from build123d import *

# Parameters (mm, degrees)
SKETCH_1_R      = 4
SKETCH_1_R_2    = 1.5
SKETCH_1_R_3    = 2
EXTRUDE_1_DEPTH = 2
SKETCH_2_R      = 1.5
EXTRUDE_2_DEPTH = 2
FILLET_2_R      = 2
SKETCH_3_R      = 2
EXTRUDE_3_DEPTH = 2
FILLET_3_R      = 2
FILLET_4_R      = 2


with BuildPart() as part:
    # 草图1 → 凸台-拉伸1 (new body)
    with BuildSketch(Plane.XY):
        with BuildLine():
            Line((-17, 18.75), (17, 18.75))
            ThreePointArc((17, 18.75), (18.414213562, 18.164213562), (19, 16.75))
            Line((19, 16.75), (19, 6.838490702))
            Line((19, 6.838490702), (20, 6.838490702))
            Line((20, 6.838490702), (20, 9.75))
            Line((20, 9.75), (27, 9.75))
            Line((27, 9.75), (29, 9.75))
            Line((29, 9.75), (29, 7.75))
            Line((29, 7.75), (29, -9.12411328))
            ThreePointArc((29, -9.12411328), (28.414213562, -10.538326843), (27, -11.12411328))
            Line((27, -11.12411328), (20, -11.12411328))
            Line((20, -11.12411328), (20, -16.75))
            Line((20, -16.75), (20, -18.75))
            Line((20, -18.75), (18, -18.75))
            Line((18, -18.75), (-18, -18.75))
            Line((-18, -18.75), (-20, -18.75))
            Line((-20, -18.75), (-20, -16.75))
            Line((-20, -16.75), (-20, -11.12411328))
            Line((-20, -11.12411328), (-27, -11.12411328))
            ThreePointArc((-27, -11.12411328), (-28.414213562, -10.538326843), (-29, -9.12411328))
            Line((-29, -9.12411328), (-29, 7.75))
            Line((-29, 7.75), (-29, 9.75))
            Line((-29, 9.75), (-27, 9.75))
            Line((-27, 9.75), (-20, 9.75))
            Line((-20, 9.75), (-20, 6.838490702))
            Line((-20, 6.838490702), (-19, 6.838490702))
            Line((-19, 6.838490702), (-19, 16.75))
            ThreePointArc((-19, 16.75), (-18.414213562, 18.164213562), (-17, 18.75))
        make_face()
        with Locations((0, -6.75)):
            Circle(SKETCH_1_R, mode=Mode.SUBTRACT)
        with Locations((-10.5, 3.75)):
            Circle(SKETCH_1_R, mode=Mode.SUBTRACT)
        with Locations((-7, -6.75)):
            Circle(SKETCH_1_R_2, mode=Mode.SUBTRACT)
        with Locations((0, 0.25)):
            Circle(SKETCH_1_R_2, mode=Mode.SUBTRACT)
        with Locations((7, -6.75)):
            Circle(SKETCH_1_R_2, mode=Mode.SUBTRACT)
        with Locations((0, -13.75)):
            Circle(SKETCH_1_R_2, mode=Mode.SUBTRACT)
        with Locations((-17.5, 3.75)):
            Circle(SKETCH_1_R_2, mode=Mode.SUBTRACT)
        with Locations((10.5, -3.25)):
            Circle(SKETCH_1_R_2, mode=Mode.SUBTRACT)
        with Locations((-10.5, 10.75)):
            Circle(SKETCH_1_R_2, mode=Mode.SUBTRACT)
        with Locations((-3.5, 3.75)):
            Circle(SKETCH_1_R_2, mode=Mode.SUBTRACT)
        with Locations((-10.5, -3.25)):
            Circle(SKETCH_1_R_2, mode=Mode.SUBTRACT)
        with Locations((17.5, 3.75)):
            Circle(SKETCH_1_R_2, mode=Mode.SUBTRACT)
        with Locations((3.5, 3.75)):
            Circle(SKETCH_1_R_2, mode=Mode.SUBTRACT)
        with Locations((10.5, 3.75)):
            Circle(SKETCH_1_R, mode=Mode.SUBTRACT)
        with Locations((10.5, 10.75)):
            Circle(SKETCH_1_R_2, mode=Mode.SUBTRACT)
        with Locations((-24.315, -6.25)):
            Circle(SKETCH_1_R_3, mode=Mode.SUBTRACT)
        with Locations((-24.315, 3.75)):
            Circle(SKETCH_1_R_3, mode=Mode.SUBTRACT)
        with Locations((24.315, 3.75)):
            Circle(SKETCH_1_R_3, mode=Mode.SUBTRACT)
        with Locations((24.315, -6.25)):
            Circle(SKETCH_1_R_3, mode=Mode.SUBTRACT)
    extrude(amount=EXTRUDE_1_DEPTH)

    # 草图2 → 凸台-拉伸2 (add)
    with BuildSketch(Plane.XZ.offset(18.75)):
        with BuildLine():
            Line((-20, 0), (20, 0))
            Line((20, 0), (20, 25))
            ThreePointArc((20, 25), (19.414213562, 26.414213562), (18, 27))
            Line((18, 27), (-18, 27))
            ThreePointArc((-18, 27), (-19.414213562, 26.414213562), (-20, 25))
            Line((-20, 25), (-20, 0))
        make_face()
        with Locations((9.7, 14)):
            Circle(SKETCH_2_R, mode=Mode.SUBTRACT)
        with Locations((-9.7, 14)):
            Circle(SKETCH_2_R, mode=Mode.SUBTRACT)
        with Locations((-2.7, 14)):
            Circle(SKETCH_2_R, mode=Mode.SUBTRACT)
        with Locations((16.7, 14)):
            Circle(SKETCH_2_R, mode=Mode.SUBTRACT)
        with Locations((9.7, 7)):
            Circle(SKETCH_2_R, mode=Mode.SUBTRACT)
        with Locations((2.7, 14)):
            Circle(SKETCH_2_R, mode=Mode.SUBTRACT)
        with Locations((9.7, 21)):
            Circle(SKETCH_2_R, mode=Mode.SUBTRACT)
        with Locations((-9.7, 7)):
            Circle(SKETCH_2_R, mode=Mode.SUBTRACT)
        with Locations((-16.7, 14)):
            Circle(SKETCH_2_R, mode=Mode.SUBTRACT)
        with Locations((-9.7, 21)):
            Circle(SKETCH_2_R, mode=Mode.SUBTRACT)
    extrude(amount=EXTRUDE_2_DEPTH)

    # 圆角2
    fillet_2_edges = [part.edges().sort_by_distance(p)[0] for p in [
        (0, -20.75, 0),
    ]]
    fillet(fillet_2_edges, radius=FILLET_2_R)

    # 草图3 → 凸台-拉伸3 (add)
    with BuildSketch(Plane(origin=(0, 9.75, 0), x_dir=(1, 0, 0), z_dir=(0, 1, 0))):
        with BuildLine():
            Line((29, 0), (20, 0))
            Line((20, 0), (20, -25))
            ThreePointArc((20, -25), (20.585786438, -26.414213562), (22, -27))
            Line((22, -27), (27, -27))
            ThreePointArc((27, -27), (28.414213562, -26.414213562), (29, -25))
            Line((29, -25), (29, 0))
        make_face()
        with Locations((24.315, -9)):
            Circle(SKETCH_3_R, mode=Mode.SUBTRACT)
        with Locations((24.315, -19)):
            Circle(SKETCH_3_R, mode=Mode.SUBTRACT)
        with BuildLine():
            Line((-29, 0), (-20, 0))
            Line((-20, 0), (-20, -25))
            ThreePointArc((-20, -25), (-20.585786438, -26.414213562), (-22, -27))
            Line((-22, -27), (-27, -27))
            ThreePointArc((-27, -27), (-28.414213562, -26.414213562), (-29, -25))
            Line((-29, -25), (-29, 0))
        make_face()
        with Locations((-24.315, -19)):
            Circle(SKETCH_3_R, mode=Mode.SUBTRACT)
        with Locations((-24.315, -9)):
            Circle(SKETCH_3_R, mode=Mode.SUBTRACT)
    extrude(amount=EXTRUDE_3_DEPTH)

    # 圆角3
    fillet_3_edges = [part.edges().sort_by_distance(p)[0] for p in [
        (24.5, 11.75, 0),
    ]]
    fillet(fillet_3_edges, radius=FILLET_3_R)

    # 圆角4
    fillet_4_edges = [part.edges().sort_by_distance(p)[0] for p in [
        (-24.5, 11.75, 0),
    ]]
    fillet(fillet_4_edges, radius=FILLET_4_R)


solid = part.part
Verification items for the finished model (mm, model axes). A direction names the side the tool comes from. Round coordinates to 2 decimals unless told otherwise and drop trailing zeros. Write each loop counter-clockwise with the first axis right and the second up, starting at its lowest first coordinate (ties: lowest second). Pieces come first, ordered by that corner, then holes.
(1) Depth check by flat-ended pin: pin 1 Ø2.5 at (x, z) = (-26, 18) entering from +Y; pin 2 Ø3.5 at (x, z) = (9.7, 21) entering from +Y; pin 3 Ø7.5 at (y, z) = (-17, 15.5) entering from +X. Enter the tip coordinate at first touch or a pass-through.
Returned:
pin 1: stops at y = 11.75
pin 2: stops at y = -18.75
pin 3: stops at x = 20
(2) Access from +Z, -Z, +X, -X, +Y, -Y to the whole of each face (thin tool, end or side, straight path). Record for faces 4 (the flat face through (20, -19, 11)), 5 (the cylindrical face through (26.223, 10.736, 8.399)).
Returned:
face 4: +Z, -Z, +X, -Y
face 5: +Y, -Y
(3) Section check C-C (z = 9.75). Enter the section's corners in (x, y).
Returned:
outline: (-29, 9.75) - (-26.17, 9.75) - (-26.17, 11.75) - (-29, 11.75) - close; (-22.46, 9.75) - (-20, 9.75) - (-20, 11.75) - (-22.46, 11.75) - close; (-20, -20.75) - (20, -20.75) - (20, -18.75) - (-20, -18.75) - close; (20, 9.75) - (22.46, 9.75) - (22.46, 11.75) - (20, 11.75) - close; (26.17, 9.75) - (29, 9.75) - (29, 11.75) - (26.17, 11.75) - close
(4) Section check A-A (z = 14). Give the number of separate pieces and of enclosed holes in the cut face, plus the area to 3 significant figures.
Returned:
separate pieces: 9
enclosed holes: 0
area: 80.0 mm2
(5) Material ranges on line 1 (X direction, y = 10, z = 18.75); line 2 (Y direction, x = 7, z = 0.8); line 3 (X direction, y = 11, z = 20), recorded low to high.
Returned:
line 1: x = -29 to -26.3, -22.33 to -20, 20 to 22.33, 26.3 to 29
line 2: y = -20.35 to -8.25, -5.25 to 1.81, 5.69 to 18.75
line 3: x = -29 to -26.05, -22.58 to -20, 20 to 22.58, 26.05 to 29
(6) Mould release check, pull along X, two halves, no side actions. Record for faces 1 (the flat face through (-24, 9.75, 14)), 2 (the cylindrical face through (28.4, 10.74, 26.43)), 3 (the cylindrical face through (25.39, 10.736, 17.314)): pulls with the +X half, pulls with the -X half, needs draft (parallel to the pull), parting line crosses it, or undercut.
Returned:
face 1: needs draft
face 2: pulls with the +X half
face 3: undercut
(7) Section check B-B (x = 7.5). Enter the section's corners in (y, z).
Returned:
outline: (-20.75, 2) arc R2 ccw to (-18.75, 0) - (-8.16, 0) - (-8.16, 2) - (-18.75, 2) - (-18.75, 27) - (-20.75, 27) - close; (-5.34, 0) - (1.1, 0) - (1.1, 2) - (-5.34, 2) - close; (6.4, 0) - (18.75, 0) - (18.75, 2) - (6.4, 2) - close
